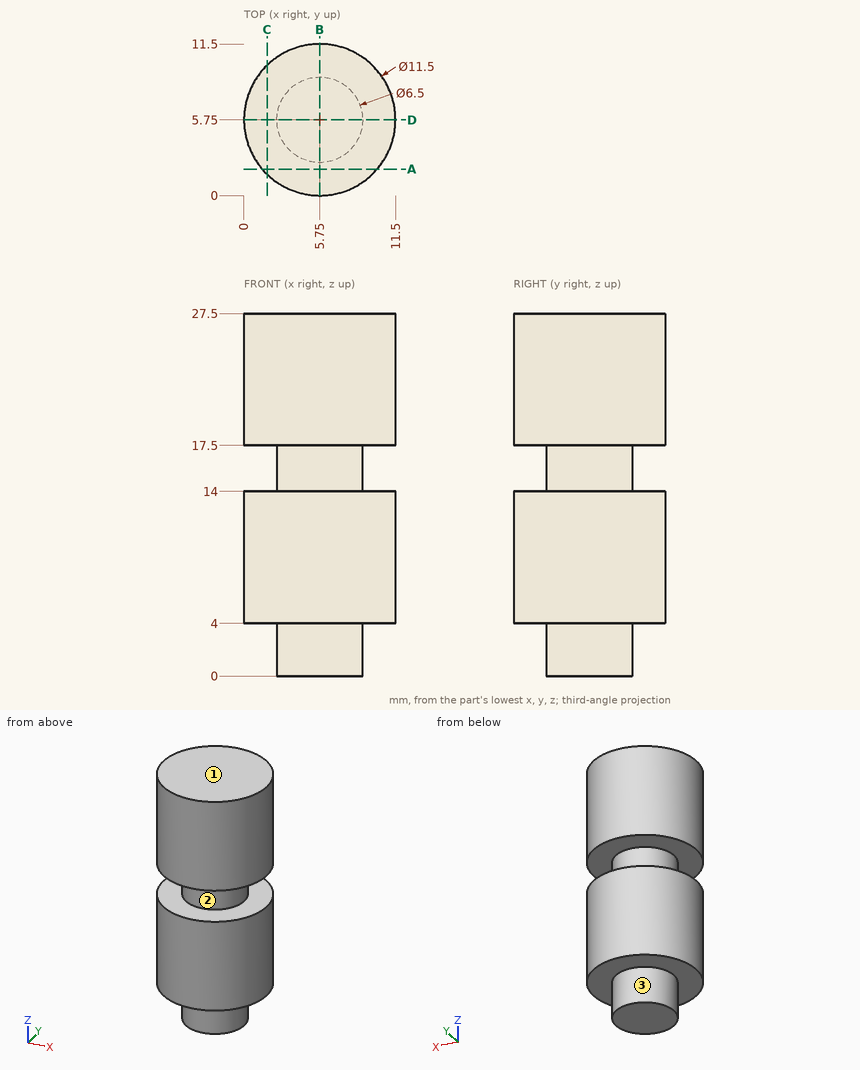
Study the drawing (mm; zero at the part's minimum x, y, z) and answer. A direction names the side the tool comes from. Give positions to 0.01 mm unless a question says otherwise; leave off trailing zeros. Loops run counter-clockwise (first coordinate to the right, second up) from the corner with the lowest first, then second, coordinate; pieces in that order, holes last. Notation, with made-up numbers: M -14,50 L 14,50 A25 cw 14,73 Z; hole C 54,-19.75 d11. An arc over 180 degrees is marked long. Use CSV: the item, a comma, the result in double quotes.
1) Find section C-C on x = 1.75. Write down the section's boundary in (y, z), plus the area to 3 significant figures.
Answer:
outline,"M 1.62,4 L 9.88,4 L 9.88,14 L 1.62,14 Z; M 1.62,17.5 L 9.88,17.5 L 9.88,27.5 L 1.62,27.5 Z"
area,"165 mm^2"
2) Find section B-B on x = 5.75. Write down the section's boundary in (y, z).
Answer:
outline,"M 0,4 L 2.5,4 L 2.5,0 L 9,0 L 9,4 L 11.5,4 L 11.5,14 L 9,14 L 9,17.5 L 11.5,17.5 L 11.5,27.5 L 0,27.5 L 0,17.5 L 2.5,17.5 L 2.5,14 L 0,14 Z"
3) Consider L1, parallel to Z at x = 6, y = 2; L2, parallel to X at y = 2, z = 26; L3, parallel to X at y = 5, z = 16.25. Determine where each line is inside the solid, lowest interval first.
Answer:
L1,"4 to 14, 17.5 to 27.5"
L2,"1.39 to 10.11"
L3,"2.59 to 8.91"
4) Find section A-A on y = 2. Write down the section's boundary in (x, z).
Answer:
outline,"M 1.39,4 L 10.11,4 L 10.11,14 L 1.39,14 Z; M 1.39,17.5 L 10.11,17.5 L 10.11,27.5 L 1.39,27.5 Z"
5) Given P1, Ø3, axis at x = 9, z = 10, coming from the -Y side; P2, Ø3, axis at x = 9.5, z = 5, coming from the -Y side; P3, Ø6, axis at x = 2.5, z = 21.5, coming from the +Y side, each flat-ended and moving along its own axis, determine where each tip first touches the part or whether it passes through.
Answer:
P1,"y = 0.27"
P2,"y = 0.46"
P3,"y = 11.49"
6) Which of the six approach directions +Z, -Z, +X, -X, +Y, -Y give full straight-line access (tool end or side, diameter ignored) to the marked faces 1, 2 and 3?
Answer:
face 1,"+Z, +X, -X, +Y, -Y"
face 2,"none"
face 3,"-Z"
